Check sheet for the modelled part. Datum: model origin and axes. Units: mm. A direction names the side the tool comes from. Coordinates: 2 decimals unless noted, no trailing zeros. Order: outer loops, then holes, each group sorted by start corner. A loop starts at its lowest first (then second) coordinate and runs counter-clockwise, first axis right, second up.
1. Set-up check for faces 1 (the cylindrical face through (4.32, 17.08, -19.35)), 2 (the flat face through (9.525, 0, 0)): record each of +Z, -Z, +X, -X, +Y, -Y from which the full face is reachable in a straight line by a thin tool's end or side.
2. Thickness scan on line 1 (Y direction, x = 4.5, z = 21); line 2 (Y direction, x = 7, z = 5); line 3 (X direction, y = 19.05, z = -16) (3 decimals). Record the ranges inside material, lowest first.
3. Cross-section at D-D (z = 0). Enter the section's corners in (x, y) (3 decimals).
4. Gauge pin test, flat end, axial feed: pin 1 Ø2.5 at (x, y) = (4.76, 19.05) entering from -Z. Record the tip position at first contact, or that the pin passes through.
5. Cross-section at C-C (z = 21). Enter the section's corners in (x, y) (3 decimals).
6. Cross-section at A-A (z = -21). Count the separate pieces of the cut face and the enclosed holes in it, then the cut area to 3 significant figures.
7. Draft check along Z on faces 3 (the flat face through (5, 0, -25.4)), 4 (the cylindrical face through (4.696, 18.526, -0.827)), 5 (the flat face through (5, 25.4, 0)). Enter one of: released by +Z, released by -Z, zero draft, split by the parting line, or undercut.
8. Cross-section at B-B (y = -13.97). Enter the section's corners in (x, z) (3 decimals).
```python
from build123d import *

# Parameters (mm, degrees)
SKETCH1_W                          = 50.8
SKETCH1_H                          = 50.8
BOSS_EXTRUDE1_DEPTH                = 9.525
F_7_16_0_4375_DIAMETER_HOLE1_D     = 11.1125
F_7_16_0_4375_DIAMETER_HOLE1_DEPTH = 70.104
F_7_16_0_4375_DIAMETER_HOLE1_TIP   = 3.338531814
F_1_2_0_5_DIAMETER_HOLE2_D         = 12.7
F_1_2_0_5_DIAMETER_HOLE2_DEPTH     = 70.104
F_1_2_0_5_DIAMETER_HOLE2_TIP       = 3.815464931
F_4_40_TAPPED_HOLE1_D              = 2.2606
F_10_32_TAPPED_HOLE1_D             = 4.0386
F_10_32_TAPPED_HOLE1_DEPTH         = 11.938
F_10_32_TAPPED_HOLE1_TIP           = 1.213317848


with BuildPart() as part:
    # Sketch1 → Boss-Extrude1 (new body)
    with BuildSketch(Plane(origin=(0, 0, 0), x_dir=(0, 0, -1), z_dir=(1, 0, 0))):
        Rectangle(SKETCH1_W, SKETCH1_H)
    extrude(amount=BOSS_EXTRUDE1_DEPTH)

    # 7/16 (0.4375) Diameter Hole1
    with Locations(Plane(origin=(9.525, 0, 0), x_dir=(0, 0, -1), z_dir=(1, 0, 0))):
        with Locations((0, -13.97)):
            Hole(F_7_16_0_4375_DIAMETER_HOLE1_D / 2, depth=F_7_16_0_4375_DIAMETER_HOLE1_DEPTH)
            with Locations((0, 0, -(F_7_16_0_4375_DIAMETER_HOLE1_DEPTH + F_7_16_0_4375_DIAMETER_HOLE1_TIP / 2))):  # 118° drill point
                Cone(0, F_7_16_0_4375_DIAMETER_HOLE1_D / 2, F_7_16_0_4375_DIAMETER_HOLE1_TIP, mode=Mode.SUBTRACT)

    # 1/2 (0.5) Diameter Hole2
    with Locations(Plane(origin=(9.525, 0, 0), x_dir=(0, 0, -1), z_dir=(1, 0, 0))):
        with Locations((0, 12.2301)):
            Hole(F_1_2_0_5_DIAMETER_HOLE2_D / 2, depth=F_1_2_0_5_DIAMETER_HOLE2_DEPTH)
            with Locations((0, 0, -(F_1_2_0_5_DIAMETER_HOLE2_DEPTH + F_1_2_0_5_DIAMETER_HOLE2_TIP / 2))):  # 118° drill point
                Cone(0, F_1_2_0_5_DIAMETER_HOLE2_D / 2, F_1_2_0_5_DIAMETER_HOLE2_TIP, mode=Mode.SUBTRACT)

    # #4-40 Tapped Hole1 (through all)
    with Locations(Plane(origin=(9.525, 0, 0), x_dir=(0, 0, -1), z_dir=(1, 0, 0))):
        with Locations((21, 12.2301), (-21, 11.74145915)):
            Hole(F_4_40_TAPPED_HOLE1_D / 2)

    # #10-32 Tapped Hole1
    with Locations(Plane(origin=(-0.669296778, 7.980106856, -25.4), x_dir=(-1, 0, 0), z_dir=(0, 0, -1))):
        with Locations((-5.431796778, -27.030106856), (-5.431796778, 11.069893144)):
            Hole(F_10_32_TAPPED_HOLE1_D / 2, depth=F_10_32_TAPPED_HOLE1_DEPTH)
            with Locations((0, 0, -(F_10_32_TAPPED_HOLE1_DEPTH + F_10_32_TAPPED_HOLE1_TIP / 2))):  # 118° drill point
                Cone(0, F_10_32_TAPPED_HOLE1_D / 2, F_10_32_TAPPED_HOLE1_TIP, mode=Mode.SUBTRACT)


solid = part.part
```
Data:
1. face 1: -Z
1. face 2: +Z, -Z, +X, +Y, -Y
2. line 1: y = -25.4 to 10.61, 12.87 to 25.4
2. line 2: y = -25.4 to -16.39, -11.55 to 8.32, 16.14 to 25.4
2. line 3: x = 0 to 2.743, 6.782 to 9.525
3. outline: (0, -25.4) - (9.525, -25.4) - (9.525, -19.526) - (0, -19.526) - close; (0, -8.414) - (9.525, -8.414) - (9.525, 5.88) - (0, 5.88) - close; (0, 18.58) - (9.525, 18.58) - (9.525, 25.4) - (0, 25.4) - close
4. pin 1: stops at z = -13
5. outline: (0, -25.4) - (9.525, -25.4) - (9.525, 10.611) - (0, 10.611) - close; (0, 12.872) - (9.525, 12.872) - (9.525, 25.4) - (0, 25.4) - close
6. separate pieces: 2
6. enclosed holes: 2
6. area: 437 mm2
7. face 3: released by -Z
7. face 4: undercut
7. face 5: zero draft
8. outline: (0, -25.4) - (9.525, -25.4) - (9.525, -5.556) - (0, -5.556) - close; (0, 5.556) - (9.525, 5.556) - (9.525, 25.4) - (0, 25.4) - close
